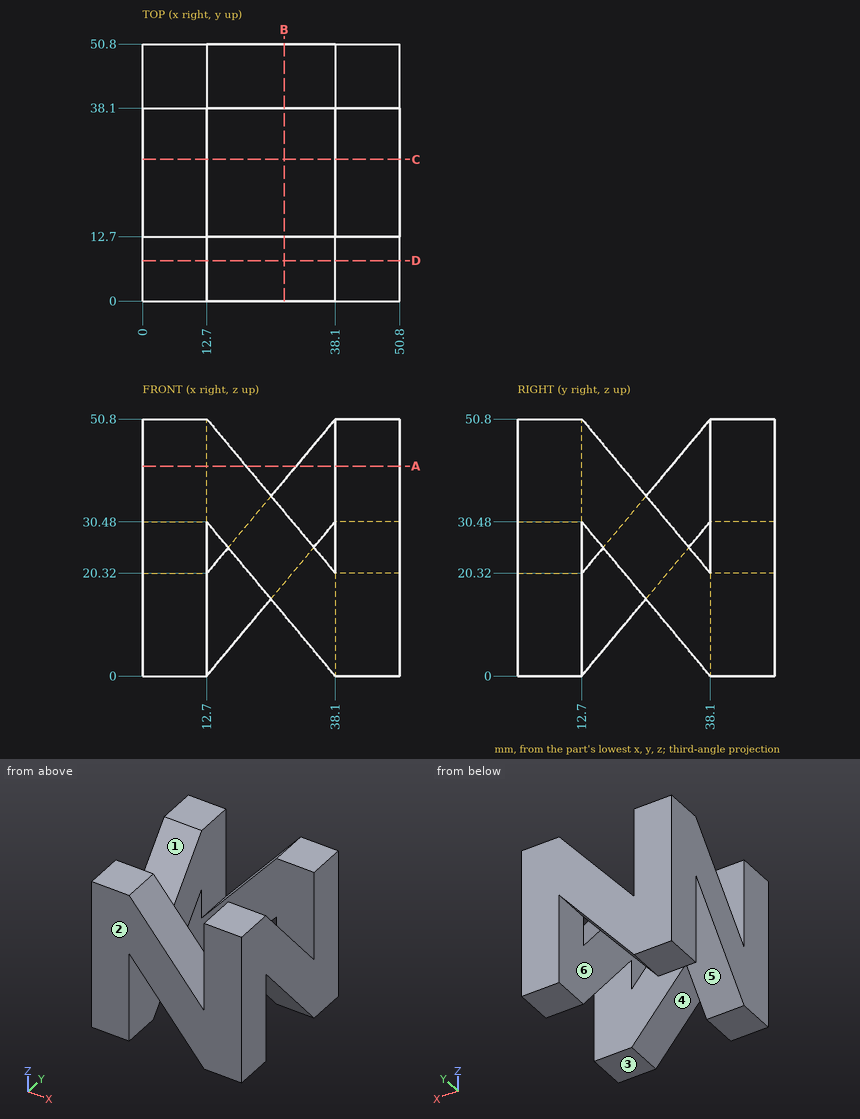
Design review of the part shown in the three views and the two pictorial views. Dimensions are in mm from the part's minimum x, y and z. A direction names the side the tool comes from. Round coordinates to 2 decimals unless told otherwise and drop trailing zeros. Write each loop counter-clockwise with the first axis right and the second up, starting at its lowest first coordinate (ties: lowest second). Pieces come first, ordered by that corner, then holes. Notation, with made-up numbers: M 40,77.25 L 58,77.25 A11 ccw 58,81.25 Z; hole C -33,-1.75 d10. An arc over 180 degrees is marked long. Use a Markdown table: item, result. Add a question column.
Q1. We need section B-B, the plane x = 28. State the section outline as (y, z) points, plus the area to 3 significant figures.
Q2. We need section D-D, the plane y = 8. State the section outline as (x, z) points.
Q3. To check wall thickness, follow line 1 (Y direction, x = 28, z = 31); line 2 (Y direction, x = 8, z = 5). State the ranges of each line that lie inside material, in increasing order.
Q4. Insertion check: pin 1 (1.5 mm diameter, centred on y = 13.5, z = 10, fed in from -X); pin 2 (3 mm diameter, centred on x = 27.5, y = 41, fed in from +Z). Each pin has a flat end and moves straight along its axis. Give the tip position at first contact, or say it passes through.
Q5. We need section A-A, the plane z = 41.5. State the section outline as (x, y) points, plus the area to 3 significant figures.
Q6. We need section C-C, the plane y = 28. State the section outline as (x, z) points.
Q7. The part is to be moulded in two halves that separate along Y. For the marked faces 1, 2 and 3, say which applies: pulls with the +Y half, pulls with the -Y half, needs draft (parallel to the pull), parting line crosses it, or undercut.
Q8. Machinability: for the marked faces 4, 5 and 6, which of the approach directions +Z, -Z, +X, -X, +Y, -Y give a long, thin tool a straight path to every point of the face, cutting with its end or side? Answer none if there is none.
Findings below:
| question | item | result |
|---|---|---|
| 1 | outline | M 0,12.12 L 12.7,12.12 L 12.7,32.44 L 0,32.44 Z; M 38.1,18.36 L 50.8,18.36 L 50.8,38.68 L 38.1,38.68 Z |
| 1 | area | 516 mm² |
| 2 | outline | M 0,0 L 12.7,0 L 12.7,30.48 L 38.1,0 L 50.8,0 L 50.8,50.8 L 38.1,50.8 L 38.1,20.32 L 12.7,50.8 L 0,50.8 Z |
| 3 | line 1 | y = 0 to 12.7, 38.1 to 50.8 |
| 3 | line 2 | y = 0 to 16.87, 38.1 to 50.8 |
| 4 | pin 1 | stops at x = 0 |
| 4 | pin 2 | stops at z = 39.88 |
| 5 | outline | M 0,0 L 20.45,0 L 20.45,12.7 L 0,12.7 Z; M 0,30.35 L 12.7,30.35 L 12.7,50.8 L 0,50.8 Z; M 30.35,38.1 L 50.8,38.1 L 50.8,50.8 L 30.35,50.8 Z; M 38.1,0 L 50.8,0 L 50.8,20.45 L 38.1,20.45 Z |
| 5 | area | 1,040 mm² |
| 6 | outline | M 0,18.36 L 12.7,18.36 L 12.7,38.68 L 0,38.68 Z; M 38.1,12.12 L 50.8,12.12 L 50.8,32.44 L 38.1,32.44 Z |
| 7 | face 1 | undercut |
| 7 | face 2 | pulls with the -Y half |
| 7 | face 3 | needs draft |
| 8 | face 4 | -Z, -Y |
| 8 | face 5 | -Z, -X |
| 8 | face 6 | none |
